Could you check a few things on this model? Use its own coordinates, in mm. A direction names the side the tool comes from. Round coordinates to 2 decimals unless told otherwise and drop trailing zeros. Loops run counter-clockwise (first coordinate to the right, second up) from the corner with the lowest first, then second, coordinate; pieces in that order, holes last. Notation, with made-up numbers: (44, -31.75) -> (53, -31.75) arc R11 ccw to (53, -12.75) -> close; hole circle Ø5 at (-28.5, -12). An arc over 180 degrees is marked (long way). Put each result on its own line as item: value. Start each with the question number.
1. Imagine slicing it at A-A, the plane z = 0. Please give me the cut outline in (x, y), and give its area (3 significant figures).
2. Which directions (+Z, -Z, +X, -X, +Y, -Y) give clear straight access to the entire face, cutting with the end or side of a thin tool? Please do faces 4 (the flat face through (-77.07, 55, -9)), 5 (the flat face through (-67.07, 23, 1)), 6 (the flat face through (-107.07, -49, 26)).
3. Imagine slicing it at B-B, the plane x = -59.5. Please give me the cut outline in (y, z).
4. Imagine slicing it at C-C, the plane z = -75. Please give me the cut outline in (x, y), and give its area (3 significant figures).
5. I'm going to push flat-ended pins straight in: P1, Ø8, axis at y = -68.5, z = 46.5, coming from the -X side; P2, Ø4, axis at x = -71, y = 34, coming from the -Z side; P3, Ø10, axis at x = -63.5, y = -39, coming from the -Z side. Where does each tip first touch, or does it pass through?
6. If we mould it in two halves opening along Z, with no side actions, what happens to faces 1 (the cylindrical face through (-91.86, 53.692, -11.923)), 2 (the flat face through (-76.57, -14, 67)), 3 (the cylindrical face through (-96.93, -2.64, -59.94))? For each: pulls with the +Z half, pulls with the -Z half, needs draft (parallel to the pull), parting line crosses it, or undercut.
7. Imagine slicing it at D-D, the plane y = 73. Please give me the cut outline in (x, z), and give its area (3 significant figures).
8. I need wall thicknesses on line 1 (Y direction, x = -92, z = 0); line 2 (X direction, y = -58.5, z = 15); line 3 (X direction, y = 42, z = -53). Which ranges of each line are inside material? Lowest first, please. Write a range as [from, to].
Autodesk Inventor part; units mm, degrees
ref_plane "YZ Plane" through (0, 0, 0) normal (1, 0, 0) x (0, 1, 0)
ref_plane "XZ Plane" through (0, 0, 0) normal (0, 1, 0) x (-1, 0, 0)
ref_plane "XY Plane" through (0, 0, 0) normal (0, 0, 1) x (1, 0, 0)
sketch "Sketch1" plane through (0, 0, 0) normal (0, 0, 1) x (1, 0, 0)
  line L0 (-56.5702, 22.5) -> (-56.5702, 60.6429)
  line L1 (-56.5702, 60.6429) -> (-76.5702, 67.5)
  line L2 (-76.5702, 67.5) -> (-76.5702, 90)
  line L3 (-76.5702, 90) -> (-87.0702, 90)
  line L4 (-87.0702, 90) -> (-87.0702, 60)
  line L5 (-87.0702, 60) -> (-67.0702, 53.1429)
  line L6 (-67.0702, 53.1429) -> (-67.0702, 22.5)
  line L7 (-67.0702, 22.5) -> (-56.5702, 22.5)
  line L8 (-104.4843, 0) -> (17.414, 0)
  point P0 (0, 0)
  dimension "d11" = 22.5
  dimension "d12" = 90
  dimension "d13" = 60
  dimension "d17" = 20
  dimension "d18" = 56.5702
  dimension "d24" = 22.5
  dimension "d31" = 10.5
  dimension "d32" = 10.5
  dimension "d33" = 10.5
revolve "Revolution1" add sketch "Sketch1" angle 360 about axis through (-10, 0, 0) along (1, 0, 0)
sketch "Sketch2" plane through (-76.5702, 0, 0) normal (1, 0, 0) x (0, 0, -1)
  circle A0 centre (0, 0) radius 67.5
  circle A1 centre (0, 0) radius 75 construction
  circle A2 centre (-75, 0) radius 7.5
  circle A3 centre (75, 0) radius 7.5
  dimension "d21" = 150
  dimension "d22" = 15
  dimension "d23" = 15
extrude "Extrusion1" cut sketch "Sketch2" against normal through all contours A2 | A3
sketch "Sketch3" plane through (-87.0702, 0, 0) normal (-1, 0, 0) x (0, 0, 1)
  circle A0 centre (0, 0) radius 60.6429
  circle A1 centre (0, 0) radius 60
  circle A2 centre (0, 0) radius 55
  dimension "d27" = 120
  dimension "d28" = 110
extrude "Extrusion2" add sketch "Sketch3" along normal mid plane 20 contours A1
sketch "Sketch4" plane through (-97.0702, 0, 0) normal (-1, 0, 0) x (0, 0, 1)
  circle A0 centre (0, 0) radius 55
  circle A1 centre (0, 0) radius 60
  dimension "d34" = 110
  dimension "d35" = 120
extrude "Extrusion3" add sketch "Sketch4" along normal blind 10
properties part number "Cover"
Entries:
1. outline: (-107.07, -60) -> (-87.07, -60) -> (-87.07, -90) -> (-76.57, -90) -> (-76.57, -67.5) -> (-56.57, -60.64) -> (-56.57, -22.5) -> (-67.07, -22.5) -> (-67.07, -53.14) -> (-77.07, -56.57) -> (-77.07, -55) -> (-107.07, -55) -> close; (-107.07, 55) -> (-77.07, 55) -> (-77.07, 56.57) -> (-67.07, 53.14) -> (-67.07, 22.5) -> (-56.57, 22.5) -> (-56.57, 60.64) -> (-76.57, 67.5) -> (-76.57, 90) -> (-87.07, 90) -> (-87.07, 60) -> (-107.07, 60) -> close
1. area: 1,980 mm^2
2. face 4: none
2. face 5: -X
2. face 6: +Z, -Z, -X, +Y, -Y
3. outline: circle Ø123.29 at (0, 0); hole circle Ø45 at (0, 0)
4. outline: (-87.07, -49.75) -> (-76.57, -49.75) -> (-76.57, -7.5) -> (-87.07, -7.5) -> close; (-87.07, 7.5) -> (-76.57, 7.5) -> (-76.57, 49.75) -> (-87.07, 49.75) -> close
4. area: 887 mm^2
5. P1: x = -87.07
5. P2: z = -57.5
5. P3: z = -53.65
6. face 1: undercut
6. face 2: needs draft
6. face 3: parting line crosses it
7. outline: (-87.07, -52.64) -> (-76.57, -52.64) -> (-76.57, 52.64) -> (-87.07, 52.64) -> close
7. area: 1,110 mm^2
8. line 1: [-60, -55], [55, 60]
8. line 2: [-87.07, -56.57]
8. line 3: [-87.07, -76.57]
